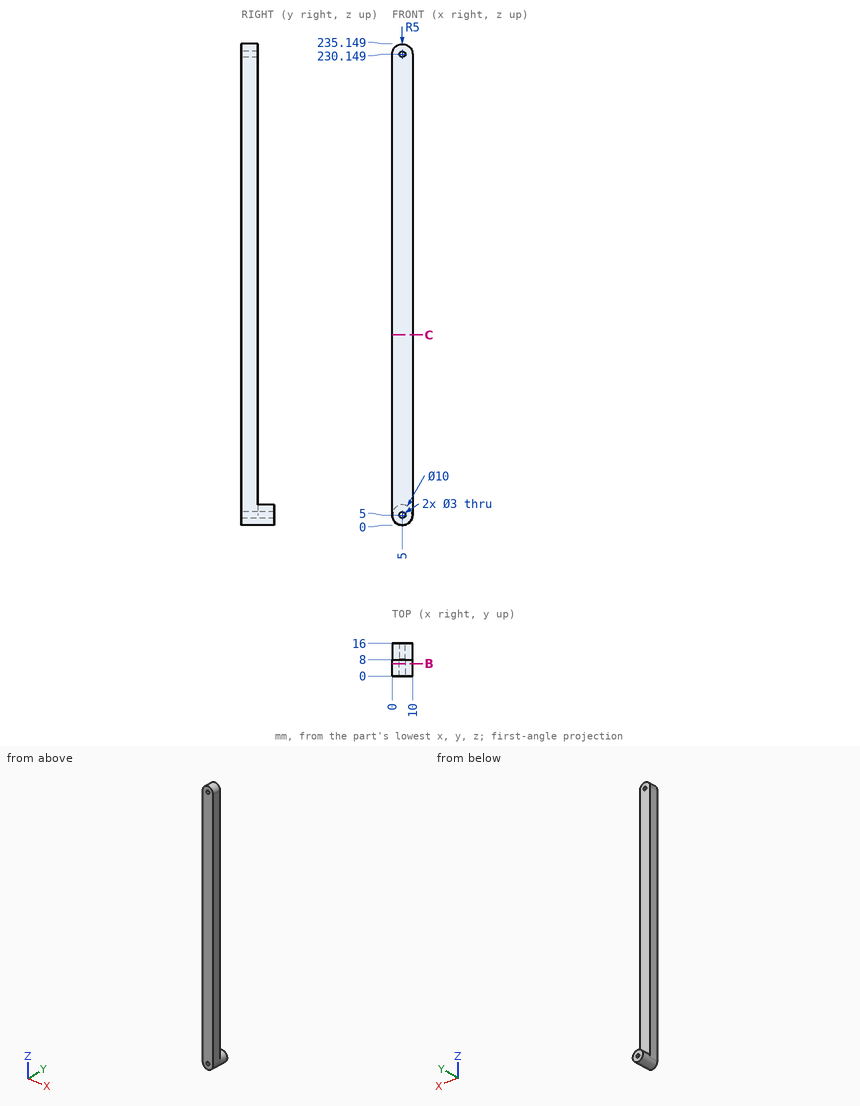
The figure shows three views and two pictorial views of one solid part (mm, origin at its lowest corner). Answer the questions. Round coordinates to 2 decimals unless told otherwise and drop trailing zeros. Order: outer loops, then holes, each group sorted by start corner. A loop starts at its lowest first (then second) coordinate and runs counter-clockwise, first axis right, second up. Notation, with made-up numbers: (50, -14.5) - (78, -14.5) arc R25 ccw to (78, 14.5) - close; hole circle Ø1 at (80, 52.25). An arc over 180 degrees is marked (long way). Write item = value, one per line. Start each with the question number.
1) Straight lines are drawn through the part: L1, parallel to Z at x = 5, y = 2.75; L2, parallel to Z at x = 5, y = 10; L3, parallel to Y at x = 9, z = 173.5. For each, find the intervals that lie inside material, in ascending order.
2) Section B-B, the plane y = 6 is taken. Write down the section's boundary in (x, z), plus the area to 3 significant figures.
3) Section C-C, the plane z = 93 is taken. Write down the section's boundary in (x, y), plus the area to 3 significant figures.
4) Given pin 1 (1.5 mm diameter, centred on x = 4.5, y = 2, fed in from -Z); pin 2 (3 mm diameter, centred on x = 4, y = 13, fed in from +Z); pin 3 (2 mm diameter, centred on x = 2.5, y = 11.5, fed in from +Z), each flat-ended and moving along its own axis, determine where each tip first touches the part or whether it passes through.
Results list:
q1.L1 = 0 to 3.5, 6.5 to 228.65, 231.65 to 235.15
q1.L2 = 0 to 3.5, 6.5 to 10
q1.L3 = 0 to 8
q2.outline = (0, 5) arc R5 ccw to (10, 5) - (10, 230.15) arc R5 ccw to (0, 230.15) - close; hole circle Ø3 at (5, 5); hole circle Ø3 at (5, 230.15)
q2.area = 2,320 mm^2
q3.outline = (0, 0) - (10, 0) - (10, 8) - (0, 8) - close
q3.area = 80.0 mm^2
q4.pin_1 = 0
q4.pin_2 = 10
q4.pin_3 = 9.77
